Model file for the job. Use its own axes, mm. Face numbers are marked on the shaded views. A direction names the side the tool comes from. Round coordinates to 2 decimals unless told otherwise and drop trailing zeros. Loops run counter-clockwise (first coordinate to the right, second up) from the corner with the lowest first, then second, coordinate; pieces in that order, holes last. Notation, with made-up numbers: (46, -39) -> (60, -39) arc R12 ccw to (60, -19) -> close; hole circle Ø7 at (-10.5, 57). An arc over 180 degrees is marked (long way). Use a Markdown table: item, result.
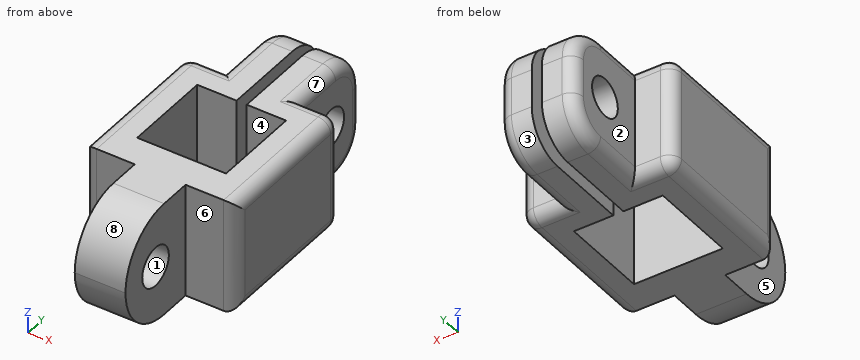
from build123d import *

# Parameters (mm, degrees)
SKETCH_1_W          = 3
SKETCH_1_H          = 7
SKETCH_1_W_2        = 12
SKETCH_1_H_2        = 12
SKETCH_1_W_3        = 7
SKETCH_1_W_4        = 5
EXTRUDE_1_DEPTH     = 9
CUT_EXTRUDE_1_DEPTH = 17.911534525
FILLET_2_R          = 3
SKETCH_4_R          = 1.5
CUT_EXTRUDE_3_DEPTH = 19.193405399
FILLET_3_R          = 1
FILLET_4_R          = 1
FILLET_5_R          = 1
SKETCH_5_W          = 5
SKETCH_5_H          = 7
CUT_EXTRUDE_4_DEPTH = 9
EXTRUDE_2_DEPTH     = 7
FILLET_6_R          = 4.5
SKETCH_7_R          = 1.55
CUT_EXTRUDE_5_DEPTH = 4


# Some blends are built 0.0001 mm under size
with BuildPart() as part:
    # 草图1 → 凸台-拉伸1 (new body)
    # profile 1 of 4: a face of its own
    with BuildSketch(Plane.XY):
        with Locations((-1.5, 9.5)):
            Rectangle(SKETCH_1_W, SKETCH_1_H)
    # profile 2 of 4: a face of its own
    with BuildSketch(Plane.XY):
        with Locations((1.5, 9.5)):
            Rectangle(SKETCH_1_W, SKETCH_1_H)
    # profile 3 of 4: a face of its own
    with BuildSketch(Plane.XY):
        Rectangle(SKETCH_1_W_2, SKETCH_1_H_2)
        Rectangle(SKETCH_1_W_3, SKETCH_1_H, mode=Mode.SUBTRACT)
    # profile 4 of 4: a face of its own
    with BuildSketch(Plane.XY):
        with Locations((1, -9.5)):
            Rectangle(SKETCH_1_W_4, SKETCH_1_H)
    extrude(amount=EXTRUDE_1_DEPTH)

    # 草图2 → 切除-拉伸1 (cut, through all)
    with BuildSketch(Plane.XY.offset(9)):
        Polygon((0, 13), (0.4, 13), (0.4, 3.5), (0, 3.5), (-0.4, 3.5), (-0.4, 13), align=None)
    extrude(amount=-CUT_EXTRUDE_1_DEPTH, mode=Mode.SUBTRACT)

    # 圆角2
    fillet_2_edges = [part.edges().sort_by_distance(p)[0] for p in [
        (1.7, 13, 9),
        (1.7, 13, 0),
        (-1.7, 13, 0),
        (-1.7, 13, 9),
    ]]
    fillet(fillet_2_edges, radius=FILLET_2_R)

    # 草图4 → 切除-拉伸3 (cut, through all)
    with BuildSketch(Plane(origin=(3, 0, 0), x_dir=(0, 0, -1), z_dir=(1, 0, 0))):
        with Locations((-4.5, 9.5)):
            Circle(SKETCH_4_R)
    extrude(amount=-CUT_EXTRUDE_3_DEPTH, mode=Mode.SUBTRACT)

    # 圆角3
    fillet_3_edges = [part.edges().sort_by_distance(p)[0] for p in [
        (3, 8, 9),
        (6, 0, 0),
        (3, 8, 0),
        (4.5, 6, 0),
        (6, 6, 4.5),
        (6, -6, 4.5),
        (4.5, 6, 9),
        (6, 0, 9),
        (3, 13, 4.5),
        (3, 12.121320344, 8.121320344),
        (3, 12.121320344, 0.878679656),
    ]]
    fillet(fillet_3_edges, radius=FILLET_3_R)

    # 圆角4
    fillet_4_edges = [part.edges().sort_by_distance(p)[0] for p in [
        (-3, 8, 9),
        (-6, 0, 0),
        (-4.5, 6, 0),
        (-3, 8, 0),
        (-4.5, 6, 9),
        (-6, 0, 9),
        (-6, -6, 4.5),
        (-3, 13, 4.5),
        (-3, 12.121320344, 8.121320344),
        (-3, 12.121320344, 0.878679656),
    ]]
    fillet(fillet_4_edges, radius=FILLET_4_R)

    # 圆角5
    # the kernel refuses this fillet: 1 mm, written as the material it takes off along each edge
    with BuildSketch(Plane(origin=(-5, 5, 8), x_dir=(0, 1, 0), z_dir=(-1, 0, 0))) as fillet_5_piece_1_section:
        Polygon((0, 0), (FILLET_5_R, 0), (FILLET_5_R, -FILLET_5_R), (0, -FILLET_5_R), align=None)
    fillet_5_piece_1 = extrude(amount=FILLET_5_R, mode=Mode.PRIVATE)
    fillet_5_piece_1 = fillet_5_piece_1 - Plane(origin=(-5, 5, 8), x_dir=(0, -0.7071067811865475, -0.7071067811865475), z_dir=(-1, 0, 0)) * Sphere(FILLET_5_R, mode=Mode.PRIVATE)
    add(fillet_5_piece_1, mode=Mode.SUBTRACT)
    with BuildSketch(Plane(origin=(-5, 5, 1), x_dir=(0, 1, 0), z_dir=(-1, 0, 0))) as fillet_5_piece_2_section:
        Polygon((0, 0), (FILLET_5_R, 0), (FILLET_5_R, FILLET_5_R), (0, FILLET_5_R), align=None)
    fillet_5_piece_2 = extrude(amount=FILLET_5_R, mode=Mode.PRIVATE)
    fillet_5_piece_2 = fillet_5_piece_2 - Plane(origin=(-5, 5, 1), x_dir=(0, -0.7071067811865475, 0.7071067811865475), z_dir=(-1, 0, 0)) * Sphere(FILLET_5_R, mode=Mode.PRIVATE)
    add(fillet_5_piece_2, mode=Mode.SUBTRACT)
    with BuildSketch(Plane(origin=(-6, 6, 1), x_dir=(0, -1, 0), z_dir=(0, 0, 1))) as fillet_5_piece_3:
        with BuildLine():
            CenterArc((FILLET_5_R, FILLET_5_R), FILLET_5_R, 180, 90)
            Line((0, FILLET_5_R), (0, 0))
            Line((0, 0), (FILLET_5_R, 0))
        make_face()
    extrude(amount=7, mode=Mode.SUBTRACT)

    # 草图5 → 切除-拉伸4 (cut)
    with BuildSketch(Plane.XY.offset(9)):
        with Locations((1, -9.5)):
            Rectangle(SKETCH_5_W, SKETCH_5_H)
    extrude(amount=-CUT_EXTRUDE_4_DEPTH, mode=Mode.SUBTRACT)

    # 草图6 → 凸台-拉伸2 (add)
    with BuildSketch(Plane.XZ.offset(6)):
        Polygon((0, 9), (-2, 9), (-2, 0), (0, 0), (2, 0), (2, 9), align=None)
    extrude(amount=EXTRUDE_2_DEPTH)

    # 圆角6
    fillet_6_edges = [part.edges().sort_by_distance(p)[0] for p in [
        (0, -13, 0),
        (0, -13, 9),
    ]]
    fillet(fillet_6_edges, radius=FILLET_6_R - 0.0001)  # a hair under: the kernel refuses the full size

    # 草图7 → 切除-拉伸5 (cut)
    with BuildSketch(Plane.ZY.offset(2)):
        with Locations((4.5, -9.5)):
            Circle(SKETCH_7_R)
    extrude(amount=-CUT_EXTRUDE_5_DEPTH, mode=Mode.SUBTRACT)


solid = part.part
Q1. Drill centre lines: L1, parallel to Y at x = 1.65, z = 4.5; L2, parallel to X at y = 3.25, z = 2.25; L3, parallel to X at y = 11.25, z = 2.5. Where is each one in solid material? Low to high. Write a range as from..to.
Results list:
| item | result |
|---|---|
| L1 | y = -13..-11.05, -7.95..-3.5, 3.5..8, 11..13 |
| L2 | x = -6..-3.5, 3.5..6 |
| L3 | x = -3..-0.4, 0.4..3 |
Q2. Tool access for the marked faces 4, 5, 6, 7 and 8: list every direction of +Z, -Z, +X, -X, +Y, -Y with a clear straight run to the whole face (end or side of a thin tool).
Results list:
| item | result |
|---|---|
| face 4 | +Z, -Z |
| face 5 | +Z, -Z, -X, -Y |
| face 6 | +Z, -Z, +X, -Y |
| face 7 | +Z, +X, +Y |
| face 8 | +Z, +X, -X, -Y |
Q3. Flat gauge pins, fed straight in: pin 1 (2 mm diameter, centred on y = -11, z = 2.5, fed in from -X); pin 2 (1.6 mm diameter, centred on x = 1.5, z = 6.5, fed in from -Y); pin 3 (0.9 mm diameter, centred on x = -3.5, z = 5.5, fed in from -Y); pin 4 (1.8 mm diameter, centred on y = 9.5, z = 4.5, fed in from +X). Where does each tip first touch, or does it go through?
Results list:
| item | result |
|---|---|
| pin 1 | stops at x = -2 |
| pin 2 | stops at y = -12.84 |
| pin 3 | stops at y = -6 |
| pin 4 | passes through |
Q4. Band-saw the part on A-A, the plane y = 9.5. Give the cut face in (x, z), plus the area to 3 significant figures.
Results list:
| item | result |
|---|---|
| outline | (-3, 1) arc R1 ccw to (-2, 0) -> (-0.4, 0) -> (-0.4, 3) -> (-3, 3) -> close; (-3, 6) -> (-0.4, 6) -> (-0.4, 9) -> (-2, 9) arc R1 ccw to (-3, 8) -> close; (0.4, 0) -> (2, 0) arc R1 ccw to (3, 1) -> (3, 3) -> (0.4, 3) -> close; (0.4, 6) -> (3, 6) -> (3, 8) arc R1 ccw to (2, 9) -> (0.4, 9) -> close |
| area | 30.3 mm² |
Q5. Band-saw the part on D-D, the plane z = 3.5. Give the number of separate pieces and of enclosed holes in the cut face, plus the area to 3 significant figures.
Results list:
| item | result |
|---|---|
| separate pieces | 4 |
| enclosed holes | 0 |
| area | 135 mm² |
Q6. Band-saw the part on C-C, the plane y = -9.5. Give the cut face in (x, z), plus the area to 3 significant figures.
Results list:
| item | result |
|---|---|
| outline | (-2, 0.11) -> (2, 0.11) -> (2, 2.95) -> (-2, 2.95) -> close; (-2, 6.05) -> (2, 6.05) -> (2, 8.89) -> (-2, 8.89) -> close |
| area | 22.7 mm² |
Q7. Band-saw the part on B-B, the plane x = 2.5. Give the cut face in (y, z), plus the area to 3 significant figures.
Results list:
| item | result |
|---|---|
| outline | (-6, 0) -> (-3.5, 0) -> (-3.5, 9) -> (-6, 9) -> close; (3.5, 0) -> (5, 0) arc R1 ccw to (5.5, 0.13) -> (10, 0.13) arc R2.87 ccw to (12.87, 3) -> (12.87, 6) arc R2.87 ccw to (10, 8.87) -> (5.5, 8.87) arc R1 ccw to (5, 9) -> (3.5, 9) -> close; hole circle Ø3 at (9.5, 4.5) |
| area | 94.2 mm² |
Q8. Pull direction Z, two halves, no side cores. Call the marked faces 1, 2 and 3: released by +Z, released by -Z, zero draft, split by the parting line, or undercut.
Results list:
| item | result |
|---|---|
| face 1 | undercut |
| face 2 | zero draft |
| face 3 | released by -Z |
